Can you work these out from the model? Positions are in its coordinate system, mm. Give positions to 0.01 mm unless a question says otherwise; leave off trailing zeros. Order: outer loops, then holes, each group sorted by start corner. A loop starts at its lowest first (then second) coordinate and runs counter-clockwise, first axis right, second up. Notation, with made-up numbers: (-18, 5) - (-9, 5) arc R33 ccw to (-9, 43) - close; hole circle Ø4 at (18, -36.5). An arc over 180 degrees is marked (long way). Return JSON: item names as keys, results as strings.
```python
from build123d import *

# Parameters (mm, degrees)
F0_R      = 6.4
F1_DEPTH  = 25.5
F3_D      = 5.1
F4_R      = 6.4
F4_R_2    = 2.55
F5_DEPTH  = 136.5
F6_SIZE2  = 1
F6_SIZE   = 1
F7_R      = 2.7297634072
F8_DEPTH  = 7
F9_R      = 3.4275534108
F10_DEPTH = 5


with BuildPart() as f1:
    # F0 (on Right) → F1 (new body)
    with BuildSketch(Plane.YZ):
        Circle(F0_R)
    extrude(amount=-F1_DEPTH)

    # F3 (through all)
    with Locations(Plane.YZ):
        with Locations((0, 0)):
            Hole(F3_D / 2)

    # F4 (on face) → F5 (join)
    with BuildSketch(Plane(origin=(-25.5, 0, 0), x_dir=(0, -1, 0), z_dir=(-1, 0, 0))):
        Circle(F4_R)
        Circle(F4_R_2, mode=Mode.SUBTRACT)
        Circle(F4_R_2)
    extrude(amount=F5_DEPTH)

    # F6
    f6_edges = [f1.edges().sort_by_distance(p)[0] for p in [
        (0, -6.4, 0),
        (-12.75, 6.4, 0),
        (-25.5, 0, -6.4),
        (-25.5, 0, 6.4),
        (-93.75, -6.4, 0),
        (-162, 6.4, 0),
    ]]
    chamfer(f6_edges, length=F6_SIZE, length2=F6_SIZE2)

    # F7 (on face) → F8 (join)
    with BuildSketch(Plane(origin=(-162, 0, 0), x_dir=(0, -1, 0), z_dir=(-1, 0, 0))):
        Circle(F7_R)
    extrude(amount=F8_DEPTH)

    # F9 (on face) → F10 (join)
    with BuildSketch(Plane(origin=(-169, 0, 0), x_dir=(0, -1, 0), z_dir=(-1, 0, 0))):
        Circle(F9_R)
    extrude(amount=-F10_DEPTH)


solid = f1.part
```
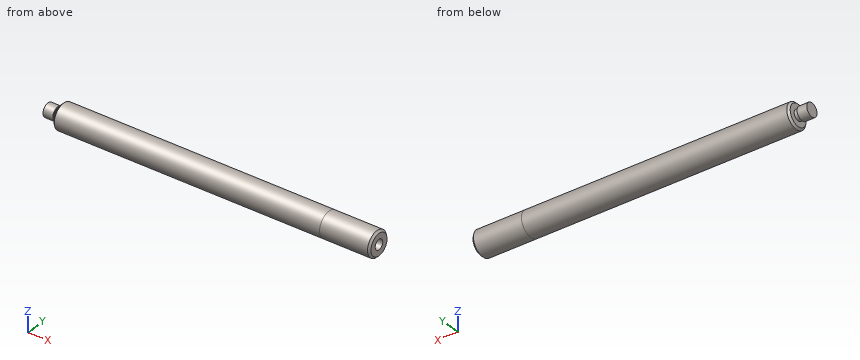
1. Suppose I cut it at A-A (y = 0). List the corners of the cut face in (x, z) for me.
Checks:
{"outline": "(-169, -3.43) - (-164, -3.43) - (-164, -2.73) - (-162, -2.73) - (-162, -5.4) - (-161, -6.4) - (-1, -6.4) - (0, -5.4) - (0, -2.55) - (-25.5, -2.55) - (-25.5, 2.55) - (0, 2.55) - (0, 5.4) - (-1, 6.4) - (-161, 6.4) - (-162, 5.4) - (-162, 2.73) - (-164, 2.73) - (-164, 3.43) - (-169, 3.43) - close"}
2. For pin 1 Ø1.5 at (x, y) = (-80.5, 1) entering from +Z; pin 2 Ø1.5 at (y, z) = (0.5, 0.5) entering from +X; pin 3 Ø3 at (x, z) = (-51, 1) entering from -Y, each with a flat end and sliding along its axis, tell me the tip position at first contact or that it passes through.
Checks:
{"pin 1": "z = 6.4", "pin 2": "x = -25.5", "pin 3": "y = -6.4"}
3. If I drill on L1, parallel to Z at x = -15.75, y = 0; L2, parallel to X at y = 1.25, z = 2.5; L3, parallel to Y at x = -32.5, z = 0.5, over which ranges is the centre line in solid material (lowest first)? Write a range as [from, to].
Checks:
{"L1": "[-6.4, -2.55], [2.55, 6.4]", "L2": "[-169, -164], [-162, 0]", "L3": "[-6.38, 6.38]"}
4. Suppose I cut it at D-D (x = -123). List the corners of the cut face in (y, z) for me, plus the area to 3 significant figures.
Checks:
{"outline": "circle Ø12.8 at (0, 0)", "area": "129 mm^2"}
5. Suppose I cut it at C-C (x = -20.5). List the corners of the cut face in (y, z) for me.
Checks:
{"outline": "circle Ø12.8 at (0, 0); hole circle Ø5.1 at (0, 0)"}
